```python
from build123d import *

# Parameters (mm, degrees)
SKETCH1_R               = 7.925
EXTRUDE1_DEPTH          = 16.84375
CUT_EXTRUDE1_DEPTH      = 21.231736556
CUT_EXTRUDE1_DEPTH_BACK = 21.231736556
SKETCH2_W               = 7.925
SKETCH2_H               = 17
SKETCH3_R               = 11
CUT_EXTRUDE2_DEPTH      = 3.5
SKETCH6_R               = 9
CUT_EXTRUDE5_DEPTH      = 4
SKETCH7_R               = 6
SKETCH7_R_2             = 1.5
CUT_EXTRUDE6_DEPTH      = 21.231736717


with BuildPart() as part:
    # Sketch1 → Extrude1 (new body)
    with BuildSketch(Plane.XY):
        Circle(SKETCH1_R)
    extrude(amount=EXTRUDE1_DEPTH)

    # Sketch2 → Cut-Extrude1 (cut, two sides: drawn at the far end of the back side and taken through both)
    with BuildSketch(Plane(origin=(0, 0, 0), x_dir=(1, 0, 0), z_dir=(0, 1, 0)).offset(-CUT_EXTRUDE1_DEPTH_BACK)):
        with Locations((3.9625, -8.5)):
            Rectangle(SKETCH2_W, SKETCH2_H)
    extrude(amount=CUT_EXTRUDE1_DEPTH + CUT_EXTRUDE1_DEPTH_BACK, mode=Mode.SUBTRACT)

    # Sketch3 → Cut-Extrude2 (cut)
    with BuildSketch(Plane(origin=(0, 0, 0), x_dir=(0, 0, -1), z_dir=(1, 0, 0))):
        with Locations((-16.873106172, 0)):
            Circle(SKETCH3_R)
    extrude(amount=-CUT_EXTRUDE2_DEPTH, mode=Mode.SUBTRACT)

    # Sketch6 → Cut-Extrude5 (cut)
    with BuildSketch(Plane(origin=(0, 0, 0), x_dir=(0, 0, -1), z_dir=(1, 0, 0))):
        with Locations((-16.84375, 0)):
            Circle(SKETCH6_R)
    extrude(amount=-CUT_EXTRUDE5_DEPTH, mode=Mode.SUBTRACT)

    # Sketch7 → Cut-Extrude6 (cut, through all)
    with BuildSketch(Plane(origin=(0, 0, 0), x_dir=(0, 0, -1), z_dir=(1, 0, 0))):
        with Locations((-16.84375, 0)):
            Circle(SKETCH7_R)
        with Locations((-3.0625, 0)):
            Circle(SKETCH7_R_2)
    extrude(amount=-CUT_EXTRUDE6_DEPTH, mode=Mode.SUBTRACT)


solid = part.part
```
Geometry check sheet. Reference: the model listing, model coordinates, mm. A direction names the side the tool comes from. Coordinates: 2 decimals unless noted, no trailing zeros. Write each loop counter-clockwise with the first axis right and the second up, starting at its lowest first coordinate (ties: lowest second). Pieces come first, ordered by that corner, then holes. Notation, with made-up numbers: M 9,55.25 L 29,55.25 A20 ccw 29,74.25 Z; hole C -30.5,32 d8. An arc over 180 degrees is marked long. Use one line per item in the form item = value. Start each with the question number.
1) Thickness scan on probe 1 along Z at (x, y) = (-1.75, 0); probe 2 along X at (y, z) = (0.25, 1); probe 3 along Z at (x, y) = (-7.25, -0.5). Record the ranges inside material, lowest first. Write a range as from..to.
2) Section check A-A on y = 0. Enter the section's corners in (x, z) (1 decimal), and give its area (3 significant figures).
3) Go/stop test with flat-tipped pins: pin 1 Ø4 at (x, z) = (-7, 11.5) entering from -Y; pin 2 Ø3.5 at (y, z) = (0, 3.06) entering from +X; pin 3 Ø2.5 at (y, z) = (1.5, 8.5) entering from +X; pin 4 Ø2.5 at (y, z) = (-3, 12.5) entering from +X. Record where each tip stops, or that it passes through.
4) Release check for a two-part mould opening along Z. For faces 1 (the flat face through (-3, 0, 0)), 2 (the cylindrical face through (-3.91, 0.45, 1.63)), 3 (the flat face through (-4.5, 6.3, 16.844)) record: pulls with the +Z half, pulls with the -Z half, needs draft (parallel to the pull), parting line crosses it, or undercut.
5) Section check C-C on x = -2.5. Enter the section's corners in (y, z).
6) Set-up check for faces 4 (the cylindrical face through (-3.746, -0.115, 7.844)), 5 (the cylindrical face through (-5.499, -0.132, 10.845)): record each of +Z, -Z, +X, -X, +Y, -Y from which the full face is reachable in a straight line by a thin tool's end or side.
7) Section check D-D on y = 2.25. Enter the section's corners in (x, z).
8) Section check B-B on z = 15. Enter the section's corners in (x, y) (3 decimals), and give its area (3 significant figures).
Responses:
q1.probe_1 = 0..1.56, 4.56..5.87
q1.probe_2 = -7.92..0
q1.probe_3 = 0..1.65, 4.48..10.86
q2.outline = M -7.9,0 L 0,0 L 0,1.6 L -7.9,1.6 Z; M -7.9,4.6 L 0,4.6 L 0,5.9 L -3.5,5.9 L -3.5,7.8 L -4,7.8 L -4,10.8 L -7.9,10.8 Z
q2.area = 43.3 mm2
q3.pin_1 = -6.15
q3.pin_2 = 0
q3.pin_3 = -3.5
q3.pin_4 = -4
q4.face_1 = pulls with the -Z half
q4.face_2 = undercut
q4.face_3 = pulls with the +Z half
q5.outline = M -7.52,0 L 7.52,0 L 7.52,8.85 A11 cw -7.52,8.85 Z; hole C 0,3.06 d3
q6.face_4 = +Z, +X
q6.face_5 = +Z, +X, -X
q7.outline = M -7.6,0 L 0,0 L 0,6.11 L -3.5,6.11 L -3.5,8.13 L -4,8.13 L -4,11.28 L -7.6,11.28 Z
q8.outline = M -5.496,-5.71 A7.925 ccw -4,-6.841 L -4,-5.71 Z; M -5.496,5.71 L -4,5.71 L -4,6.841 A7.925 ccw Z
q8.area = 1.83 mm2
